Autodesk Inventor part; units mm, degrees
ref_plane "YZ Plane" through (0, 0, 0) normal (1, 0, 0) x (0, 1, 0)
ref_plane "XZ Plane" through (0, 0, 0) normal (0, 1, 0) x (-1, 0, 0)
ref_plane "XY Plane" through (0, 0, 0) normal (0, 0, 1) x (1, 0, 0)
sketch "Sketch1" plane through (0, 0, 0) normal (0, 0, 1) x (1, 0, 0)
  line L0 (-34.8609, 0) -> (34.8609, 0) construction
  line L1 (0, -34.8609) -> (0, 34.8609) construction
  line L2 (0, 0) -> (11.6542, 11.6542) construction
  line L3 (0, 0) -> (16.4815, 0) construction
  line L4 (0, 24.9006) -> (16.8, 24.9006)
  line L5 (16.8, 24.9006) -> (16.8, 21.2406)
  line L6 (16.8, 21.2406) -> (19.0203, 19.0203)
  line L7 (24.9006, 0) -> (24.9006, 16.8)
  line L8 (24.9006, 16.8) -> (21.2406, 16.8)
  line L9 (21.2406, 16.8) -> (19.0203, 19.0203)
  line L10 (0, 0) -> (-11.6542, 11.6542) construction
  line L11 (0, 0) -> (-16.4815, 0) construction
  line L12 (0, 24.9006) -> (-16.8, 24.9006)
  line L13 (-16.8, 24.9006) -> (-16.8, 21.2406)
  line L14 (-16.8, 21.2406) -> (-19.0203, 19.0203)
  line L15 (-24.9006, 0) -> (-24.9006, 16.8)
  line L16 (-24.9006, 16.8) -> (-21.2406, 16.8)
  line L17 (-21.2406, 16.8) -> (-19.0203, 19.0203)
  line L18 (0, 0) -> (11.6542, -11.6542) construction
  line L19 (0, -24.9006) -> (16.8, -24.9006)
  line L20 (16.8, -24.9006) -> (16.8, -21.2406)
  line L21 (16.8, -21.2406) -> (19.0203, -19.0203)
  line L22 (24.9006, 0) -> (24.9006, -16.8)
  line L23 (24.9006, -16.8) -> (21.2406, -16.8)
  line L24 (21.2406, -16.8) -> (19.0203, -19.0203)
  line L25 (0, 0) -> (-11.6542, -11.6542) construction
  line L26 (0, -24.9006) -> (-16.8, -24.9006)
  line L27 (-16.8, -24.9006) -> (-16.8, -21.2406)
  line L28 (-16.8, -21.2406) -> (-19.0203, -19.0203)
  line L29 (-24.9006, 0) -> (-24.9006, -16.8)
  line L30 (-24.9006, -16.8) -> (-21.2406, -16.8)
  line L31 (-21.2406, -16.8) -> (-19.0203, -19.0203)
  dimension "d0" = 45
  dimension "d1" = 3.14
  dimension "d2" = 3.66
  dimension "d3" = 16.8
extrude "Extrusion1" add sketch "Sketch1" along normal blind 4
hole "Hole1" at (0, 0, 0) direction (0, 0, 1) diameter 40 end through all
sketch "Sketch6" plane through (0, 0, 4) normal (0, 0, 1) x (1, 0, 0)
  circle A0 centre (0, 0) radius 20 construction
  line L0 (16.8, 24.9006) -> (-16.8, 24.9006) construction
  line L1 (-16.8, 24.9006) -> (-16.8, 21.2406) construction
  line L2 (-16.8, 21.2406) -> (-21.2406, 16.8) construction
  line L3 (-21.2406, 16.8) -> (-24.9006, 16.8) construction
  line L4 (-24.9006, 16.8) -> (-24.9006, -16.8) construction
  line L5 (-24.9006, -16.8) -> (-21.2406, -16.8) construction
  line L6 (-21.2406, -16.8) -> (-16.8, -21.2406) construction
  line L7 (-16.8, -21.2406) -> (-16.8, -24.9006) construction
  line L8 (-16.8, -24.9006) -> (16.8, -24.9006) construction
  line L9 (16.8, -24.9006) -> (16.8, -21.2406) construction
  line L10 (16.8, -21.2406) -> (21.2406, -16.8) construction
  line L11 (21.2406, -16.8) -> (24.9006, -16.8) construction
  line L12 (24.9006, -16.8) -> (24.9006, 16.8) construction
  line L13 (24.9006, 16.8) -> (21.2406, 16.8) construction
  line L14 (21.2406, 16.8) -> (16.8, 21.2406) construction
  line L15 (16.8, 21.2406) -> (16.8, 24.9006) construction
  circle A1 centre (0, 0) radius 20
  circle A2 centre (0, 0) radius 13.5
  dimension "d42" = 40
  dimension "d43" = 27
extrude "Extrusion4" [suppressed]
sketch "Sketch8" plane through (0, 0, 4) normal (0, 0, 1) x (1, 0, 0)
  line L0 (16.8, 24.9006) -> (-16.8, 24.9006)
  line L1 (-16.8, 24.9006) -> (-16.8, 21.2406)
  line L2 (-16.8, 21.2406) -> (-21.2406, 16.8)
  line L3 (-21.2406, 16.8) -> (-24.9006, 16.8)
  line L4 (-24.9006, 16.8) -> (-24.9006, -16.8)
  line L5 (-24.9006, -16.8) -> (-21.2406, -16.8)
  line L6 (-21.2406, -16.8) -> (-16.8, -21.2406)
  line L7 (-16.8, -21.2406) -> (-16.8, -24.9006)
  line L8 (-16.8, -24.9006) -> (16.8, -24.9006)
  line L9 (16.8, -24.9006) -> (16.8, -21.2406)
  line L10 (16.8, -21.2406) -> (21.2406, -16.8)
  line L11 (21.2406, -16.8) -> (24.9006, -16.8)
  line L12 (24.9006, -16.8) -> (24.9006, 16.8)
  line L13 (24.9006, 16.8) -> (21.2406, 16.8)
  line L14 (21.2406, 16.8) -> (16.8, 21.2406)
  line L15 (16.8, 21.2406) -> (16.8, 24.9006)
  line L16 (-23.9006, -15.8) -> (-23.9006, 15.8)
  line L17 (-23.9006, 15.8) -> (-20.8264, 15.8)
  line L18 (-20.8264, 15.8) -> (-15.8, 20.8264)
  line L19 (-15.8, 20.8264) -> (-15.8, 23.9006)
  line L20 (-15.8, 23.9006) -> (15.8, 23.9006)
  line L21 (15.8, 23.9006) -> (15.8, 20.8264)
  line L22 (15.8, 20.8264) -> (20.8264, 15.8)
  line L23 (20.8264, 15.8) -> (23.9006, 15.8)
  line L24 (23.9006, 15.8) -> (23.9006, -15.8)
  line L25 (23.9006, -15.8) -> (20.8264, -15.8)
  line L26 (20.8264, -15.8) -> (15.8, -20.8264)
  line L27 (15.8, -20.8264) -> (15.8, -23.9006)
  line L28 (15.8, -23.9006) -> (-15.8, -23.9006)
  line L29 (-15.8, -23.9006) -> (-15.8, -20.8264)
  line L30 (-15.8, -20.8264) -> (-20.8264, -15.8)
  line L31 (-20.8264, -15.8) -> (-23.9006, -15.8)
  circle A0 centre (0, 0) radius 20
  circle A1 centre (0, 0) radius 19.2
  dimension "d41" = 1
  dimension "d46" = 0.8
extrude "Extrusion6" add sketch "Sketch8" against normal up to surface (4 mm away)
sketch "Sketch9" plane through (0, 0, 0) normal (0, 0, -1) x (-1, 0, 0)
  circle A0 centre (-23.1006, 15) radius 1.05
  circle A1 centre (23.1006, -15) radius 1.05
  point P0 (0, 0)
extrude "Extrusion7" cut sketch "Sketch9" against normal through all
properties part number "20_Cube_Insert_CirAp_Guide"
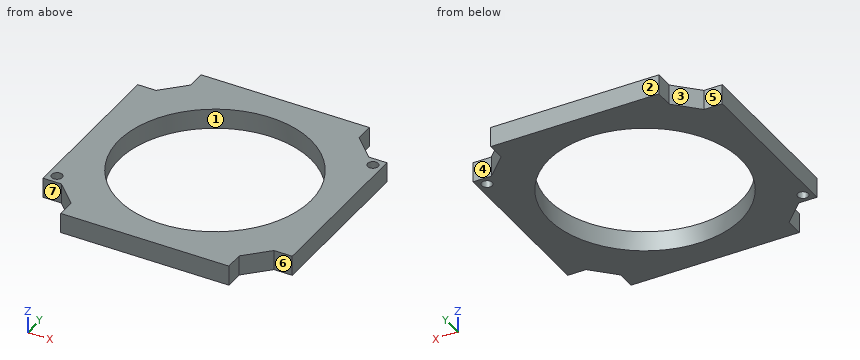
Build history of the part. All positions in model axes, mm. Face numbers are marked on the shaded views. A direction names the side the tool comes from. Coordinates: 2 decimals unless noted, no trailing zeros. Write each loop counter-clockwise with the first axis right and the second up, starting at its lowest first coordinate (ties: lowest second). Pieces come first, ordered by that corner, then holes. Notation, with made-up numbers: (54.25, 68.5) -> (66.25, 68.5) arc R18 ccw to (66.25, 96.5) -> close; hole circle Ø2 at (22, -22). An arc over 180 degrees is marked (long way). Use CSV: the item, a comma, the result in double quotes. Start each with the question number.
Q1. Drill centre lines: probe 1 along Y at (x, z) = (23, 3.3); probe 2 along X at (y, z) = (0.5, 3.2); probe 3 along Y at (x, z) = (-21.5, 0.3). Where is each one in solid material? Low to high.
Q2. Cut at C-C, the plane z = 2.15. List the corners of the cut face in (x, y).
Q3. Pull direction X, two halves, no side cores. Call the marked faces 1, 2 and 3: released by +X, released by -X, zero draft, split by the parting line, or undercut.
Q4. 3-axis set-ups, long thin cutter, end or side, ignore diameter. For the marked faces 4, 5, 6 and 7: which of +Z, -Z, +X, -X, +Y, -Y reach the whole face in a straight line?
Q5. Flat gauge pins, fed straight in: pin 1 Ø1.9 at (x, y) = (-23.1, -15) entering from -Z; pin 2 Ø1.1 at (x, z) = (-23, 2) entering from +Y; pin 3 Ø1.8 at (y, z) = (-22.5, 1) entering from -X; pin 4 Ø1.8 at (y, z) = (-23.5, 2.5) entering from +X. Where does each tip first touch, or does it go through?
Q6. Cut at A-A, the plane x = 0. List the corners of the cut face in (y, z), then the cut area to 3 significant figures.
Q7. Cut at D-D, the plane y = -15. List the corners of the cut face in (x, z) (3 decimals).
Checked values:
1,probe 1,"y = -16.8 to 13.95, 16.05 to 16.8"
1,probe 2,"x = -24.9 to -19.19, 19.19 to 24.9"
1,probe 3,"y = -16.8 to 16.8"
2,outline,"(-24.9, -16.8) -> (-21.24, -16.8) -> (-16.8, -21.24) -> (-16.8, -24.9) -> (16.8, -24.9) -> (16.8, -21.24) -> (21.24, -16.8) -> (24.9, -16.8) -> (24.9, 16.8) -> (21.24, 16.8) -> (16.8, 21.24) -> (16.8, 24.9) -> (-16.8, 24.9) -> (-16.8, 21.24) -> (-21.24, 16.8) -> (-24.9, 16.8) -> close; hole circle Ø2.1 at (-23.1, -15); hole circle Ø38.4 at (0, 0); hole circle Ø2.1 at (23.1, 15)"
3,face 1,"undercut"
3,face 2,"zero draft"
3,face 3,"released by -X"
4,face 4,"+Z, -Z, +X, +Y"
4,face 5,"+Z, -Z, -X, +Y"
4,face 6,"+Z, -Z, +X, -Y"
4,face 7,"+Z, -Z, -X, -Y"
5,pin 1,"passes through"
5,pin 2,"stops at y = 16.8"
5,pin 3,"stops at x = -16.8"
5,pin 4,"stops at x = 16.8"
6,outline,"(-24.9, 0) -> (-19.2, 0) -> (-19.2, 4) -> (-24.9, 4) -> close; (19.2, 0) -> (24.9, 0) -> (24.9, 4) -> (19.2, 4) -> close"
6,area,"45.6 mm²"
7,outline,"(-24.901, 0) -> (-24.151, 0) -> (-24.151, 4) -> (-24.901, 4) -> close; (-22.051, 0) -> (-11.985, 0) -> (-11.985, 4) -> (-22.051, 4) -> close; (11.985, 0) -> (24.901, 0) -> (24.901, 4) -> (11.985, 4) -> close"
